```python
from build123d import *

# Parameters (mm, degrees)
SKETCH1_W                   = 190.5
SKETCH1_H                   = 793.115
BOSS_EXTRUDE1_DEPTH         = 3.175
F_1_4_0_25_DIAMETER_HOLE1_D = 6.35
F_1_1_DIAMETER_SLOT1_DEPTH  = 3.175
FILLET1_R                   = 2.54


# Read off the part's stored shape, not the designer's step: 1 (1) Diameter Slot1
with BuildPart() as part:
    # Sketch1 → Boss-Extrude1 (new body)
    with BuildSketch(Plane.XY):
        with Locations((95.25, 396.5575)):
            Rectangle(SKETCH1_W, SKETCH1_H)
    extrude(amount=BOSS_EXTRUDE1_DEPTH)

    # 1/4 (0.25) Diameter Hole1 (through all)
    with Locations(Plane.XY.offset(3.175)):
        with Locations((15.875, 716.915), (15.875, 510.8575), (15.875, 282.2575), (15.875, 76.2), (174.625, 76.2), (174.625, 282.2575), (174.625, 510.8575), (174.625, 716.915)):
            Hole(F_1_4_0_25_DIAMETER_HOLE1_D / 2)

    # 1 (1) Diameter Slot1 outline → 1 (1) Diameter Slot1 (cut)
    with BuildSketch(Plane.XY):
        with BuildLine():
            Line((161.925, 691.515), (161.925, 742.315))
            ThreePointArc((161.925, 742.315), (149.225, 755.015), (136.525, 742.315))
            Line((136.525, 742.315), (136.525, 691.515))
            ThreePointArc((136.525, 691.515), (149.225, 678.815), (161.925, 691.515))
        make_face()
        with BuildLine():
            ThreePointArc((161.925, 536.2575), (149.225, 548.9575), (136.525, 536.2575))
            Line((136.525, 536.2575), (136.525, 485.4575))
            ThreePointArc((136.525, 485.4575), (149.225, 472.7575), (161.925, 485.4575))
            Line((161.925, 485.4575), (161.925, 536.2575))
        make_face()
        with BuildLine():
            ThreePointArc((161.925, 307.6575), (149.225, 320.3575), (136.525, 307.6575))
            Line((136.525, 307.6575), (136.525, 256.8575))
            ThreePointArc((136.525, 256.8575), (149.225, 244.1575), (161.925, 256.8575))
            Line((161.925, 256.8575), (161.925, 307.6575))
        make_face()
        with BuildLine():
            ThreePointArc((161.925, 101.6), (149.225, 114.3), (136.525, 101.6))
            Line((136.525, 101.6), (136.525, 50.8))
            ThreePointArc((136.525, 50.8), (149.225, 38.1), (161.925, 50.8))
            Line((161.925, 50.8), (161.925, 101.6))
        make_face()
        with BuildLine():
            Line((53.975, 50.8), (53.975, 101.6))
            ThreePointArc((53.975, 101.6), (41.275, 114.3), (28.575, 101.6))
            Line((28.575, 101.6), (28.575, 50.8))
            ThreePointArc((28.575, 50.8), (41.275, 38.1), (53.975, 50.8))
        make_face()
        with BuildLine():
            ThreePointArc((53.975, 307.6575), (41.275, 320.3575), (28.575, 307.6575))
            Line((28.575, 307.6575), (28.575, 256.8575))
            ThreePointArc((28.575, 256.8575), (41.275, 244.1575), (53.975, 256.8575))
            Line((53.975, 256.8575), (53.975, 307.6575))
        make_face()
        with BuildLine():
            ThreePointArc((53.975, 536.2575), (41.275, 548.9575), (28.575, 536.2575))
            Line((28.575, 536.2575), (28.575, 485.4575))
            ThreePointArc((28.575, 485.4575), (41.275, 472.7575), (53.975, 485.4575))
            Line((53.975, 485.4575), (53.975, 536.2575))
        make_face()
        with BuildLine():
            ThreePointArc((53.975, 742.315), (41.275, 755.015), (28.575, 742.315))
            Line((28.575, 742.315), (28.575, 691.515))
            ThreePointArc((28.575, 691.515), (41.275, 678.815), (53.975, 691.515))
            Line((53.975, 691.515), (53.975, 742.315))
        make_face()
    extrude(amount=F_1_1_DIAMETER_SLOT1_DEPTH, mode=Mode.SUBTRACT)

    # Fillet1
    fillet1_edges = [part.edges().sort_by_distance(p)[0] for p in [
        (0, 793.115, 1.5875),
        (190.5, 793.115, 1.5875),
        (190.5, 0, 1.5875),
        (0, 0, 1.5875),
    ]]
    fillet(fillet1_edges, radius=FILLET1_R)


solid = part.part
```
Geometry check sheet. Reference: the model listing, model coordinates, mm. A direction names the side the tool comes from. Give positions to 0.01 mm unless a question says otherwise; leave off trailing zeros. Loops run counter-clockwise (first coordinate to the right, second up) from the corner with the lowest first, then second, coordinate; pieces in that order, holes last. Notation, with made-up numbers: M -29,8.5 L 20,8.5 A26 ccw 20,30.5 Z; hole C 60.5,59 d11. An arc over 180 degrees is marked long. Write item = value, one per line. Start each with the question number.
1. Go/stop test with flat-tipped pins: P1, Ø10, axis at x = 174.625, y = 716.915, coming from the +Z side (3 decimals); P2, Ø5.5, axis at x = 15.88, y = 282.26, coming from the -Z side. Record where each tip stops, or that it passes through.
2. Section check B-B, the plane z = 1.3. Give the number of separate pieces and of enclosed holes in the cut face, plus the area to 3 significant figures.
3. Tool access check on faces 3 (the face through (40.996, 678.818, 1.565)), 4 (the face through (94, 402, 0)). Record the directions out of +Z, -Z, +X, -X, +Y, -Y that give a thin tool (end or side, any length) a straight path to the whole face; none if there is none.
4. Draft check along X on faces 1 (the face through (94, 402, 3.175)), 2 (the face through (41, 472.76, 1.57)). Enter one of: +X half, -X half, draft (parallel to the pull), parting line (faces both ways), or undercut.
5. Section check A-A, the plane y = 495. Enter the section's corners in (x, z) (3 decimals).
6. Thickness scan on probe 1 along X at (y, z) = (710.5, 1.9) (3 decimals); probe 2 along Y at (x, z) = (42, 1.25) (3 decimals); probe 3 along Y at (x, z) = (49, 3) (3 decimals). Record the ranges inside material, lowest first.
Values follow:
q1.P1 = 3.175
q1.P2 = through
q2.separate_pieces = 1
q2.enclosed_holes = 16
q2.area = 136,000 mm^2
q3.face_3 = +Z, -Z
q3.face_4 = -Z, +X, -X, +Y, -Y
q4.face_1 = draft
q4.face_2 = undercut
q5.outline = M 0,0 L 28.575,0 L 28.575,3.175 L 0,3.175 Z; M 53.975,0 L 136.525,0 L 136.525,3.175 L 53.975,3.175 Z; M 161.925,0 L 190.5,0 L 190.5,3.175 L 161.925,3.175 Z
q6.probe_1 = 0 to 28.575, 53.975 to 136.525, 161.925 to 190.5
q6.probe_2 = 0 to 38.121, 114.279 to 244.178, 320.337 to 472.778, 548.937 to 678.836, 754.994 to 793.115
q6.probe_3 = 0 to 40.72, 111.68 to 246.777, 317.738 to 475.377, 546.338 to 681.435, 752.395 to 793.115
